Can you work these out from the model? Positions are in its coordinate system, mm. Face numbers are marked on the shaded views. A direction names the side the tool comes from. Round coordinates to 2 decimals unless told otherwise and drop trailing zeros. Order: outer loops, then holes, each group sorted by start corner. A loop starts at its lowest first (then second) coordinate and runs counter-clockwise, first axis right, second up. Notation, with made-up numbers: M 39.5,-31 L 83.5,-31 A8 ccw 83.5,-21 Z; hole C 16.5,51.5 d7. An arc over 180 degrees is marked long. One line per question, with ' | ' between items.
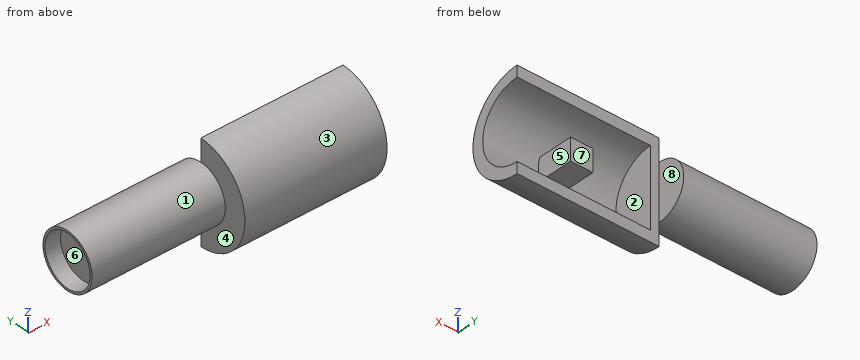
```python
from build123d import *

# Parameters (mm, degrees)
BOSS_EXTRUDE1_DEPTH      = 30
BOSS_EXTRUDE1_DEPTH_BACK = 30
BOSS_EXTRUDE2_REACH      = 46.732
BOSS_EXTRUDE2_END_RADIUS = 17.5
BOSS_EXTRUDE2_START      = -1
SKETCH3_W                = 10
SKETCH3_H                = 10
BOSS_EXTRUDE3_START      = 4
BOSS_EXTRUDE3_DEPTH      = 4
SKETCH5_R                = 12.5
BOSS_EXTRUDE4_DEPTH      = 60
SKETCH6_R                = 11.5
CUT_EXTRUDE1_DEPTH       = 7


with BuildPart() as part:
    # Sketch1 → Boss-Extrude1 (new, two sides: drawn at the far end of the back side and taken through both)
    with BuildSketch(Plane(origin=(0, 0, 0), x_dir=(0, 0, -1), z_dir=(1, 0, 0)).offset(-BOSS_EXTRUDE1_DEPTH_BACK)):
        with BuildLine():
            Line((-17.5, 0), (-22.5, 0))
            ThreePointArc((-22.5, 0), (0, -22.5), (22.5, 0))
            Line((22.5, 0), (17.5, 0))
            ThreePointArc((17.5, 0), (0, -17.5), (-17.5, 0))
        make_face()
    extrude(amount=BOSS_EXTRUDE1_DEPTH + BOSS_EXTRUDE1_DEPTH_BACK)

    # Boss-Extrude2: up to this cylinder (the profile starts inside it)
    boss_extrude2_end = Plane(origin=(0, 0, 0), z_dir=(1, 0, 0)) * Cylinder(BOSS_EXTRUDE2_END_RADIUS, 129.464, mode=Mode.PRIVATE)
    # Sketch3 → Boss-Extrude2 (add, up to the surface)
    with BuildSketch(Plane(origin=(0, 0, 0), x_dir=(1, 0, 0), z_dir=(0, 1, 0)).offset(BOSS_EXTRUDE2_START), mode=Mode.PRIVATE) as boss_extrude2_sk1:
        Rectangle(SKETCH3_W, SKETCH3_H)
    boss_extrude2_tool1 = extrude(boss_extrude2_sk1.sketch, amount=-BOSS_EXTRUDE2_REACH, mode=Mode.PRIVATE) & boss_extrude2_end
    add(boss_extrude2_tool1.solids().sort_by_distance((0, -1, 0))[0])

    # Sketch4 → Boss-Extrude3 (add)
    with BuildSketch(Plane.ZY.offset(30).offset(BOSS_EXTRUDE3_START)):
        with BuildLine():
            Line((-22.5, 0), (22.5, 0))
            ThreePointArc((22.5, 0), (0, -22.5), (-22.5, 0))
        make_face()
    extrude(amount=-BOSS_EXTRUDE3_DEPTH)

    # Sketch5 → Boss-Extrude4 (add)
    with BuildSketch(Plane.ZY.offset(34)):
        Circle(SKETCH5_R)
    extrude(amount=BOSS_EXTRUDE4_DEPTH)

    # Sketch6 → Cut-Extrude1 (cut)
    with BuildSketch(Plane.ZY.offset(94)):
        Circle(SKETCH6_R)
    extrude(amount=-CUT_EXTRUDE1_DEPTH, mode=Mode.SUBTRACT)


solid = part.part
```
(1) Will these pins go through, and if not, where does the flat tip stop? pin 1 Ø14 at (y, z) = (0, 0) entering from +X; pin 2 Ø14 at (y, z) = (9, 5) entering from +X; pin 3 Ø2 at (y, z) = (-1.5, -15.5) entering from +X.
Final values:
pin 1: x = 5 | pin 2: x = -34 | pin 3: x = -30
(2) Please list where these lines run through material, in increasing order: probe 1 along Y at (x, z) = (-90, 0); probe 2 along X at (y, z) = (-1, -12); probe 3 along X at (y, z) = (-8, 19.5). Write a range as [from, to].
Final values:
probe 1: [-12.5, -11.5], [11.5, 12.5] | probe 2: [-94, -30] | probe 3: [-34, 30]
(3) Thinking about a two-plate mould opening in Y: for the marked faces 6, 7 and 8, which applies, released by +Y, released by -Y, zero draft, split by the parting line, or undercut?
Final values:
face 6: undercut | face 7: released by +Y | face 8: zero draft
(4) If we section it at B-B on z = 0: Please give me the cut outline in (x, y).
Final values:
outline: M -94,-12.5 L -34,-12.5 L -34,-22.5 L 30,-22.5 L 30,-17.5 L 5,-17.5 L 5,-1 L -5,-1 L -5,-17.5 L -30,-17.5 L -30,0 L -34,0 L -34,12.5 L -94,12.5 L -94,11.5 L -87,11.5 L -87,-11.5 L -94,-11.5 Z
(5) On a 3-axis mill with a long thin cutter (end or side, diameter ignored), from which of +Z, -Z, +X, -X, +Y, -Y can I reach the whole of each face in a straight line? I mean the marked faces 1, 2, 3, 4 and 5. Say none if no direction works.
Final values:
face 1: -X | face 2: +Y | face 3: +X, -X, -Y | face 4: -X, -Y | face 5: +X, +Y
(6) If we section it at C-C on x = 13: Please give me the cut outline in (y, z).
Final values:
outline: M 0,-22.5 L 0,-17.5 A17.5 cw 0,17.5 L 0,22.5 A22.5 ccw Z
(7) If we section it at A-A on y = -5.5: Please give me the cut outline in (x, z), plus the area to 3 significant figures.
Final values:
outline: M -94,-11.22 L -34,-11.22 L -34,-21.82 L 30,-21.82 L 30,-16.61 L -30,-16.61 L -30,16.61 L 30,16.61 L 30,21.82 L -34,21.82 L -34,11.22 L -94,11.22 L -94,10.1 L -87,10.1 L -87,-10.1 L -94,-10.1 Z; M -5,-5 L 5,-5 L 5,5 L -5,5 Z | area: 2,100 mm^2
(8) If we section it at D-D on y = 7.5: Please give me the cut outline in (x, z), plus the area to 3 significant figures.
Final values:
outline: M -94,-10 L -34,-10 L -34,10 L -94,10 L -94,8.72 L -87,8.72 L -87,-8.72 L -94,-8.72 Z | area: 1,080 mm^2
